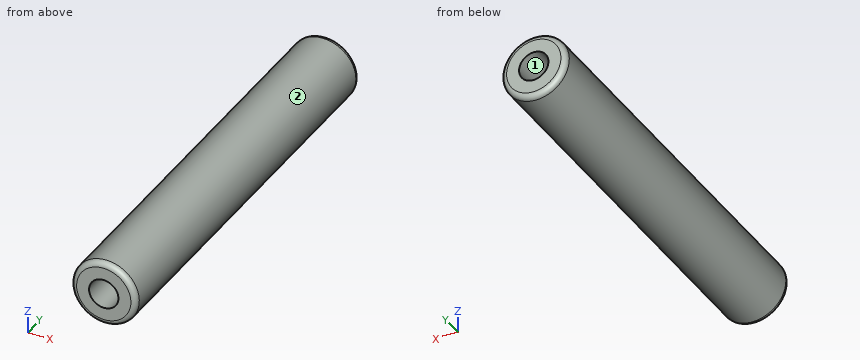
from build123d import *

# Parameters (mm, degrees)
BOSS_EXTRUDE1_DEPTH       = 18.65
BOSS_EXTRUDE1_DEPTH_BACK  = 18.65
SKETCH1_R                 = 3
F_6_32_TAPPED_HOLE1_D     = 2.7051
F_6_32_TAPPED_HOLE1_DEPTH = 12.5
F_6_32_TAPPED_HOLE1_TIP   = 0.81269403
F_6_32_TAPPED_HOLE2_D     = 2.7051
F_6_32_TAPPED_HOLE2_DEPTH = 12.5
F_6_32_TAPPED_HOLE2_TIP   = 0.81269403
FILLET1_R                 = 0.5


with BuildPart() as part:
    # Sketch1 → Boss-Extrude1 (new, two sides: drawn at the far end of the back side and taken through both)
    with BuildSketch(Plane(origin=(0, 0, 0), x_dir=(1, 0, 0), z_dir=(0, 1, 0)).offset(-BOSS_EXTRUDE1_DEPTH_BACK)):
        with Locations(Location((0, 0, 0), (0, 0, 270))):
            Circle(SKETCH1_R)
    extrude(amount=BOSS_EXTRUDE1_DEPTH + BOSS_EXTRUDE1_DEPTH_BACK)

    # 6-32 Tapped Hole1
    with Locations(Plane(origin=(0, 18.65, 0), x_dir=(1, 0, 0), z_dir=(0, 1, 0))):
        with Locations((0, 0)):
            Hole(F_6_32_TAPPED_HOLE1_D / 2, depth=F_6_32_TAPPED_HOLE1_DEPTH)
            with Locations((0, 0, -(F_6_32_TAPPED_HOLE1_DEPTH + F_6_32_TAPPED_HOLE1_TIP / 2))):  # 118° drill point
                Cone(0, F_6_32_TAPPED_HOLE1_D / 2, F_6_32_TAPPED_HOLE1_TIP, mode=Mode.SUBTRACT)

    # 6-32 Tapped Hole2
    with Locations(Plane(origin=(0, -18.65, 0), x_dir=(-1, 0, 0), z_dir=(0, -1, 0))):
        with Locations((0, 0)):
            Hole(F_6_32_TAPPED_HOLE2_D / 2, depth=F_6_32_TAPPED_HOLE2_DEPTH)
            with Locations((0, 0, -(F_6_32_TAPPED_HOLE2_DEPTH + F_6_32_TAPPED_HOLE2_TIP / 2))):  # 118° drill point
                Cone(0, F_6_32_TAPPED_HOLE2_D / 2, F_6_32_TAPPED_HOLE2_TIP, mode=Mode.SUBTRACT)

    # Fillet1
    fillet1_edges = [part.edges().sort_by_distance(p)[0] for p in [
        (0, -18.65, -3),
        (0, 18.65, -3),
    ]]
    fillet(fillet1_edges, radius=FILLET1_R)


solid = part.part
CAD build for the part. Positions are in the model's coordinates, mm. Face numbers are marked on the shaded views. Round coordinates to 2 decimals unless told otherwise and drop trailing zeros. Write each loop counter-clockwise with the first axis right and the second up, starting at its lowest first coordinate (ties: lowest second). Pieces come first, ordered by that corner, then holes. Notation, with made-up numbers: M 82.5,30.25 L 94.5,30.25 A11 cw 94.5,48.25 Z; hole C -4,13.5 d9. An arc over 180 degrees is marked long. Use a Markdown table: item, result. Add a question column.
1. Pull direction X, two halves, no side cores. Call the marked faces 1 and 2: released by +X, released by -X, zero draft, split by the parting line, or undercut.
2. Slice it at A-A on y = -14. Give the cut face in (x, z).
3. Slice it at B-B on y = 1. Give the cut face in (x, z), then the cut area to 3 significant figures.
4. Flat gauge pins, fed straight in: P1, Ø1.5, axis at x = 0.5, z = 0.5, coming from the -Y side; P2, Ø2.5, axis at x = 0, z = 0, coming from the +Y side; P3, Ø2, axis at x = 0, z = 0, coming from the -Y side. Where does each tip first touch, or does it go through?
5. Drill centre lines: probe 1 along Z at (x, y) = (1.65, 6.5); probe 2 along Z at (x, y) = (0.6, 10); probe 3 along X at (y, z) = (-13.5, -1.15). Where is each one in solid material? Low to high.
Reply:
| question | item | result |
|---|---|---|
| 1 | face 1 | undercut |
| 1 | face 2 | split by the parting line |
| 2 | outline | C 0,0 d6; hole C 0,0 d2.71 |
| 3 | outline | C 0,0 d6 |
| 3 | area | 28.3 mm^2 |
| 4 | P1 | stops at y = -18.65 |
| 4 | P2 | stops at y = 6.09 |
| 4 | P3 | stops at y = -5.94 |
| 5 | probe 1 | z = -2.51 to 2.51 |
| 5 | probe 2 | z = -2.94 to -1.21, 1.21 to 2.94 |
| 5 | probe 3 | x = -2.77 to -0.71, 0.71 to 2.77 |
